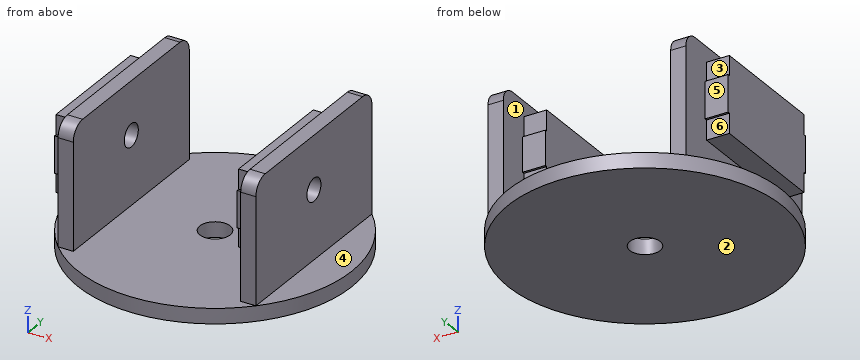
```python
from build123d import *

# Parameters (mm, degrees)
SKETCH1_R           = 90
BOSS_EXTRUDE1_DEPTH = 10
SKETCH2_W           = 10
SKETCH2_H           = 124.350526514
BOSS_EXTRUDE2_DEPTH = 80
FILLET1_R           = 10
SKETCH3_R           = 7.5
CUT_EXTRUDE1_DEPTH  = 201.616596644
SKETCH4_R           = 10
CUT_EXTRUDE2_DEPTH  = 30
BOSS_EXTRUDE5_DEPTH = 15
BOSS_EXTRUDE6_DEPTH = 15


with BuildPart() as part:
    # Sketch1 → Boss-Extrude1 (new body)
    with BuildSketch(Plane.XY):
        Circle(SKETCH1_R)
    extrude(amount=BOSS_EXTRUDE1_DEPTH)

    # Sketch2 → Boss-Extrude2 (add)
    with BuildSketch(Plane.XY.offset(10)):
        with Locations((-60.071012279, 0)):
            Rectangle(SKETCH2_W, SKETCH2_H)
        with Locations((60.071012279, 0)):
            Rectangle(SKETCH2_W, SKETCH2_H)
    extrude(amount=BOSS_EXTRUDE2_DEPTH)

    # Fillet1
    fillet1_edges = [part.edges().sort_by_distance(p)[0] for p in [
        (60.071012279, 62.175263257, 90),
        (60.071012279, -62.175263257, 90),
        (-60.071012279, 62.175263257, 90),
        (-60.071012279, -62.175263257, 90),
    ]]
    fillet(fillet1_edges, radius=FILLET1_R)

    # Sketch3 → Cut-Extrude1 (cut, through all)
    with BuildSketch(Plane.ZY.offset(65.071012279)):
        with Locations((55, 0)):
            Circle(SKETCH3_R)
    extrude(amount=-CUT_EXTRUDE1_DEPTH, mode=Mode.SUBTRACT)

    # Sketch4 → Cut-Extrude2 (cut)
    with BuildSketch(Plane.XY.offset(10)):
        Circle(SKETCH4_R)
    extrude(amount=-CUT_EXTRUDE2_DEPTH, mode=Mode.SUBTRACT)

    # Sketch7 → Boss-Extrude5 (add)
    with BuildSketch(Plane.ZY.offset(65.071012279)):
        Polygon((30, 40), (30, -40), (42.954861641, -40), (42.954861641, -41.5), (67.045138359, -41.5), (67.045138359, -40), (80, -40), (80, 40), (67.045138359, 40), (67.045138359, 41.5), (42.954861641, 41.5), (42.954861641, 40), align=None)
    extrude(amount=BOSS_EXTRUDE5_DEPTH)

    # Sketch8 → Boss-Extrude6 (add)
    with BuildSketch(Plane.ZY.offset(-55.071012279)):
        Polygon((30, 40), (30, -40), (42.954861641, -40), (42.954861641, -41.5), (67.045138359, -41.5), (67.045138359, -40), (80, -40), (80, 40), (66.344670443, 40), (66.344670443, 41.5), (43.655329557, 41.5), (43.655329557, 40), align=None)
    extrude(amount=BOSS_EXTRUDE6_DEPTH)


solid = part.part
```
Source: CAD feature listing. Evaluate the final solid. Frame: model axes, mm. Face numbers are marked on the shaded views. A direction names the side the tool comes from. Coordinates: 2 decimals unless noted, no trailing zeros. Loops run counter-clockwise (first coordinate to the right, second up) from the corner with the lowest first, then second, coordinate; pieces in that order, holes last. Notation, with made-up numbers: M 29.5,63 L 52.5,63 A19 cw 52.5,80 Z; hole C 47,28.5 d3. An arc over 180 degrees is marked long. Put each result on its own line as item: value. Start each with the question number.
1) Ray query, L1, parallel to X at y = -26.5, z = 57; L2, parallel to Z at x = -77.5, y = -25.5; L3, parallel to X at y = -53, z = 15. Return the intervals inside material, ascending. Write a range as from..to.
2) Reachability of the marked faces 4, 5 and 6 from +Z, -Z, +X, -X, +Y, -Y: full face, straight path, thin tool, end or side. Return the list, or none.
3) Contact query for flat-ended pins moving along their axis: pin 1 Ø8 at (x, z) = (60.5, 43) entering from -Y; pin 2 Ø4.5 at (y, z) = (1, 51.5) entering from +X; pin 3 Ø7.5 at (x, z) = (48.5, 53.5) entering from -Y; pin 4 Ø12 at (x, y) = (-9, -35) entering from -Z. Output: stop coordinate, or through.
4) Cut plane D-D on z = 55. Return the cut outline in (x, y).
5) Pull-direction query (Z, two-part tool) for the marked faces 1, 2 and 3; classes: pulls with the +Z half, pulls with the -Z half, needs draft (parallel to the pull), parting line crosses it, or undercut.
6) Cut plane A-A on x = 0. Return the cut outline in (y, z), then the cut area to 3 significant figures.
7) Cut plane B-B on z = 22.5. Return the cut outline in (x, y).
The answers:
1. L1: x = -80.07..-55.07, 40.07..65.07
1. L2: z = 0..10, 30..80
1. L3: x = -65.07..-55.07, 55.07..65.07
2. face 4: +Z, +X, +Y, -Y
2. face 5: +Z, -X, +Y
2. face 6: -X, +Y
3. pin 1: stops at y = -62.18
3. pin 2: stops at x = 55.07
3. pin 3: stops at y = -41.5
3. pin 4: stops at z = 0
4. outline: M -80.07,-41.5 L -65.07,-41.5 L -65.07,-62.18 L -55.07,-62.18 L -55.07,-7.5 L -65.07,-7.5 L -65.07,7.5 L -55.07,7.5 L -55.07,62.18 L -65.07,62.18 L -65.07,41.5 L -80.07,41.5 Z; M 40.07,-41.5 L 55.07,-41.5 L 55.07,-62.18 L 65.07,-62.18 L 65.07,-7.5 L 55.07,-7.5 L 55.07,7.5 L 65.07,7.5 L 65.07,62.18 L 55.07,62.18 L 55.07,41.5 L 40.07,41.5 Z
5. face 1: undercut
5. face 2: pulls with the -Z half
5. face 3: needs draft
6. outline: M -90,0 L -10,0 L -10,10 L -90,10 Z; M 10,0 L 90,0 L 90,10 L 10,10 Z
6. area: 1,600 mm²
7. outline: M -65.07,-62.18 L -55.07,-62.18 L -55.07,62.18 L -65.07,62.18 Z; M 55.07,-62.18 L 65.07,-62.18 L 65.07,62.18 L 55.07,62.18 Z
